Source: CAD feature listing. Evaluate the final solid. Frame: model axes, mm. A direction names the side the tool comes from. Round coordinates to 2 decimals unless told otherwise and drop trailing zeros. Loops run counter-clockwise (first coordinate to the right, second up) from the corner with the lowest first, then second, coordinate; pieces in that order, holes last.
Item 1: Pull-direction query (Y, two-part tool) for faces 5 (the flat face through (-101.88, 353.81, 3.82)), 6 (the flat face through (-167, 278, 8.1)), 7 (the cylindrical face through (-174.35, 284.27, 5.8)); classes: released by +Y, released by -Y, zero draft, split by the parting line, or undercut.
Item 2: Section query B-B on x = -171. Return loops of the section in (y, z), then the cut area to 3 significant figures.
Item 3: First-contact query: P1, Ø10, axis at x = -221, y = 212.5, coming from the +Z side; P2, Ø10, axis at x = -218, y = 213, coming from the -Z side; P3, Ø1.5, axis at x = -230.5, z = 7, coming from the -Y side. Flat tips, straight axial feed; report the tip coordinate or a pass-through.
Item 4: Access query for faces 1 (the flat face through (-219, 214, 8.1)), 2 (the flat face through (-194, 249, 0.4)), 3 (the flat face through (-273, 149, 0)), 4 (the flat face through (-167, 278, 1.1)). Directions: +Z, -Z, +X, -X, +Y, -Y. A direction counts if a zero-diameter tool reaches every point of the face in a straight line with its end or side. Return the directions, or none.
Item 5: Ray query, L1, parallel to Y at x = -226.5, z = 2.5; L2, parallel to Z at x = -145, y = 305.5; L3, parallel to X at y = 215, z = 5.75 (3 decimals). Return the intervals inside material, ascending.
Item 6: Section query A-A on z = 5. Return loops of the section in (x, y).
Item 7: Section query D-D on x = -124.5. Return loops of the section in (y, z).
Item 8: Section query C-C on y = 198. Return loops of the section in (x, z).
```python
from build123d import *

# Parameters (mm, degrees)
F1_DEPTH = 10
F2_DEPTH = 0.4
F4_DEPTH = 319.7
F5_R     = 10
F6_DEPTH = 8.1
F7_DEPTH = 1.1


with BuildPart() as f1:
    # F0 (on Top) → F1 (new body)
    with BuildSketch(Plane.XY):
        Polygon((-118.766080561, 367.3347540892), (-143.7718247791, 336.1143640196), (-98.9293357238, 336.1143640196), (-91.4482392501, 345.4547278984), align=None)
        Polygon((-98.9293357238, 336.1143640196), (-143.7718247791, 336.1143640196), (-179.8142472891, 291.1143640196), (-152.4964059782, 269.2343378288), align=None)
        Polygon((-152.4964059782, 269.2343378288), (-179.8142472891, 291.1143640196), (-236.384913462, 220.4842620314), (-209.0670721511, 198.6042358405), align=None)
        Polygon((-264.2086340252, 129.7584116274), (-264.2086340252, 185.7455475346), (-295.4658142978, 146.7200599476), (-268.1479729869, 124.8400337568), align=None)
        Polygon((-236.8907927142, 163.8655213438), (-264.2086340252, 185.7455475346), (-264.2086340252, 129.7584116274), align=None)
        Polygon((-236.384913462, 220.4842620314), (-264.2086340252, 185.7455475346), (-236.8907927142, 163.8655213438), (-209.0670721511, 198.6042358405), align=None)
    extrude(amount=F1_DEPTH)

    # F0 (on Top) + F1_face (on face) → F2 (cut)
    with BuildSketch(Plane.XY):
        Polygon((-98.9293357238, 336.1143640196), (-143.7718247791, 336.1143640196), (-179.8142472891, 291.1143640196), (-152.4964059782, 269.2343378288), align=None)
        Polygon((-152.4964059782, 269.2343378288), (-179.8142472891, 291.1143640196), (-236.384913462, 220.4842620314), (-209.0670721511, 198.6042358405), align=None)
        Polygon((-236.8907927142, 163.8655213438), (-264.2086340252, 185.7455475346), (-264.2086340252, 129.7584116274), align=None)
        Polygon((-236.384913462, 220.4842620314), (-264.2086340252, 185.7455475346), (-236.8907927142, 163.8655213438), (-209.0670721511, 198.6042358405), align=None)
    with BuildSketch(Plane(origin=(-193.4570267739, 246.087393923, 10), x_dir=(1, 0, 0), z_dir=(0, 0, 1))):
        Polygon((74.6909462129, 121.2473601662), (-102.0087875238, -99.3673339754), (-74.6909462129, -121.2473601662), (102.0087875238, 99.3673339754), align=None)
    extrude(amount=F2_DEPTH, mode=Mode.SUBTRACT)

    # F3 (on face) → F4 (cut)
    with BuildSketch(Plane(origin=(-43.8801592677, -54.7856395198, 0), x_dir=(0.7805097517, -0.6251436055, 0), z_dir=(-0.6251436055, -0.7805097517, 0))):
        Polygon((-322.3350566332, 0), (-287.3350566332, 10), (-322.3350566332, 10), align=None)
        Polygon((-287.3350566332, 10), (-290.9218451271, 22.5537597288), (-325.9218451271, 12.5537597288), (-322.3350566332, 0), (-322.3350566332, 10), align=None)
    extrude(amount=-F4_DEPTH, mode=Mode.SUBTRACT)

    # F5 (on Top) → F6 (join)
    with BuildSketch(Plane.XY):
        with Locations((-219.2109416958, 213.7656019243)):
            Circle(F5_R)
        with Locations((-166.8104226756, 277.7009841669)):
            Circle(F5_R)
    extrude(amount=F6_DEPTH)

    # F5 (on Top) → F7 (cut)
    with BuildSketch(Plane.XY):
        with Locations((-219.2109416958, 213.7656019243)):
            Circle(F5_R)
        with Locations((-166.8104226756, 277.7009841669)):
            Circle(F5_R)
    extrude(amount=F7_DEPTH, mode=Mode.SUBTRACT)


solid = f1.part
```
Data:
1. face 5: released by +Y
1. face 6: zero draft
1. face 7: undercut
2. outline: (246.13, 0.4) - (268.62, 0.4) - (268.62, 1.1) - (286.78, 1.1) - (286.78, 0.4) - (299.88, 0.4) - (286.78, 2.74) - (286.78, 8.1) - (268.62, 8.1) - (268.62, 5.98) - (246.13, 10) - close
2. area: 313 mm2
3. P1: stops at z = 8.1
3. P2: stops at z = 1.1
3. P3: stops at y = 170.91
4. face 1: +Z, -X, +Y
4. face 2: -Z, +X, -Y
4. face 3: -Z, +X, -X, +Y, -Y
4. face 4: -Z
5. L1: y = 176.84 to 220.61
5. L2: z = 0.4 to 5.19
5. L3: x = -229.134 to -195.935
6. outline: (-281.81, 135.78) - (-268.15, 124.84) - (-91.45, 345.45) - (-105.11, 356.39) - (-161.4, 286.11) arc R10 ccw to (-173.84, 270.58) - (-213.04, 221.64) arc R10 ccw to (-225.54, 206.03) - close
7. outline: (304.19, 0.4) - (336.11, 0.4) - (336.11, 0) - (360.18, 0) - (304.19, 10) - close
8. outline: (-252.6, 0.4) - (-209.55, 0.4) - (-209.55, 10) - close
